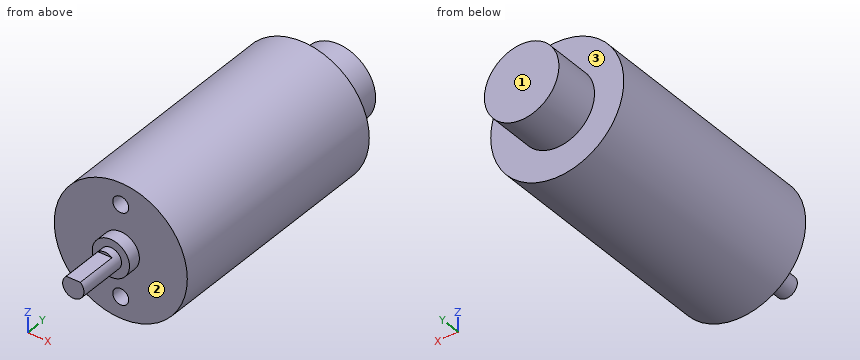
```python
from build123d import *

# Parameters (mm, degrees)
SKETCH1_R           = 12.5
BODY_DEPTH          = 46
SKETCH2_R           = 7
BOSS_EXTRUDE4_DEPTH = 9
SKETCH5_R           = 3.5
SKETCH5_R_2         = 2
BOSS_EXTRUDE5_DEPTH = 2.5
SKETCH10_R          = 2
BOSS_EXTRUDE6_DEPTH = 12
CUT_EXTRUDE1_DEPTH  = 8
SKETCH13_R          = 1.5
CUT_EXTRUDE2_DEPTH  = 4


with BuildPart() as part:
    # Sketch1 → Body (new body)
    with BuildSketch(Plane(origin=(0, 0, 0), x_dir=(1, 0, 0), z_dir=(0, 1, 0))):
        Circle(SKETCH1_R)
    extrude(amount=BODY_DEPTH)

    # Sketch2 → Boss-Extrude4 (add)
    with BuildSketch(Plane(origin=(0, 46, 0), x_dir=(1, 0, 0), z_dir=(0, 1, 0))):
        Circle(SKETCH2_R)
    extrude(amount=BOSS_EXTRUDE4_DEPTH)

    # Sketch5 → Boss-Extrude5 (add)
    with BuildSketch(Plane(origin=(0, 0, 0), x_dir=(1, 0, 0), z_dir=(0, 1, 0))):
        Circle(SKETCH5_R)
        Circle(SKETCH5_R_2, mode=Mode.SUBTRACT)
    extrude(amount=-BOSS_EXTRUDE5_DEPTH)

    # Sketch10 → Boss-Extrude6 (add)
    with BuildSketch(Plane(origin=(0, 0, 0), x_dir=(1, 0, 0), z_dir=(0, 1, 0))):
        Circle(SKETCH10_R)
    extrude(amount=-BOSS_EXTRUDE6_DEPTH)

    # Sketch12 → Cut-Extrude1 (cut)
    with BuildSketch(Plane.XZ.offset(12)):
        with BuildLine():
            Line((-1.322875656, 1.5), (1.322875656, 1.5))
            ThreePointArc((1.322875656, 1.5), (0, 2), (-1.322875656, 1.5))
        make_face()
    extrude(amount=-CUT_EXTRUDE1_DEPTH, mode=Mode.SUBTRACT)

    # Sketch13 → Cut-Extrude2 (cut)
    with BuildSketch(Plane(origin=(0, 0, 0), x_dir=(1, 0, 0), z_dir=(0, 1, 0))):
        with Locations((0, 8.5)):
            Circle(SKETCH13_R)
        with Locations((0, -8.5)):
            Circle(SKETCH13_R)
    extrude(amount=CUT_EXTRUDE2_DEPTH, mode=Mode.SUBTRACT)


solid = part.part
```
CAD build for the part. Positions are in the model's coordinates, mm. Face numbers are marked on the shaded views. A direction names the side the tool comes from. Round coordinates to 2 decimals unless told otherwise and drop trailing zeros. Order: outer loops, then holes, each group sorted by start corner. A loop starts at its lowest first (then second) coordinate and runs counter-clockwise, first axis right, second up.
Q1. Slice it at D-D (z = -8.5). Write the cut outline in (x, y).
Q2. Wall check: L1, parallel to Z at x = 0, y = 2.15; L2, parallel to Y at x = 2, z = 6.25; L3, parallel to Y at x = 9.75, z = 2. Give the ranges that are in metal, low to high.
Q3. Slice it at A-A (z = 0). Write the cut outline in (x, y), and give its area (3 significant figures).
Q4. Drop flat-ended pins along their axis: pin 1 (1 mm diameter, centred on y = 16.5, z = 9, fed in from -X); pin 2 (10 mm diameter, centred on x = 6.5, y = 17, fed in from +Z); pin 3 (3 mm diameter, centred on x = 7.5, z = -2.5, fed in from +Y); pin 4 (7.5 mm diameter, centred on x = 0.5, z = 6, fed in from -Y). Give the stop position or say it passes through.
Q5. Slice it at C-C (y = 38.5). Write the cut outline in (x, z).
Q6. Slice it at B-B (x = 0). Write the cut outline in (y, z).
Q7. Which spindle directions (+Z, -Z, +X, -X, +Y, -Y) get a long thin tool onto all of the face, cutting with end or side? Do the marked faces 1, 2 and 3. Say none if no direction does.
Results below:
1. outline: (-9.17, 0) - (-1.5, 0) - (-1.5, 4) - (1.5, 4) - (1.5, 0) - (9.17, 0) - (9.17, 46) - (-9.17, 46) - close
2. L1: z = -12.5 to -10, -7 to 7, 10 to 12.5
2. L2: y = 0 to 55
2. L3: y = 0 to 46
3. outline: (-12.5, 0) - (-3.5, 0) - (-3.5, -2.5) - (-2, -2.5) - (-2, -12) - (2, -12) - (2, -2.5) - (3.5, -2.5) - (3.5, 0) - (12.5, 0) - (12.5, 46) - (7, 46) - (7, 55) - (-7, 55) - (-7, 46) - (-12.5, 46) - close
3. area: 1,330 mm2
4. pin 1: stops at x = -9.17
4. pin 2: stops at z = 12.41
4. pin 3: stops at y = 55
4. pin 4: stops at y = -2.5
5. outline: circle Ø25 at (0, 0)
6. outline: (-12, -2) - (-2.5, -2) - (-2.5, -3.5) - (0, -3.5) - (0, -7) - (4, -7) - (4, -10) - (0, -10) - (0, -12.5) - (46, -12.5) - (46, -7) - (55, -7) - (55, 7) - (46, 7) - (46, 12.5) - (0, 12.5) - (0, 10) - (4, 10) - (4, 7) - (0, 7) - (0, 3.5) - (-2.5, 3.5) - (-2.5, 2) - (-4, 2) - (-4, 1.5) - (-12, 1.5) - close
7. face 1: +Z, -Z, +X, -X, +Y
7. face 2: -Y
7. face 3: +Y
